```python
from build123d import *

# Parameters (mm, degrees)
F1_DEPTH = 5
F3_DEPTH = 2


with BuildPart() as f1:
    # F0 (on Top) → F1 (new body)
    with BuildSketch(Plane.XY):
        Polygon((37.573822, 49.251007), (-55.58905, 49.251007), (-55.58905, -67.659264), (-31.55629, -43.860067), (37.573822, -43.860067), align=None)
    extrude(amount=F1_DEPTH)

    # F2 (on face) → F3 (cut)
    with BuildSketch(Plane.XY.offset(5)):
        Polygon((-25.10905, 34.337802), (-40.34905, 34.337802), (-40.34905, -27.690759), (-4.78905, -27.690759), (-4.78905, -12.450759), (-25.10905, -12.450759), align=None)
        Polygon((22.333822, 34.337802), (-0.526178, 34.337802), (-13.226178, 19.097802), (7.093822, 19.097802), (7.093822, -27.690759), (22.333822, -27.690759), align=None)
    extrude(amount=-F3_DEPTH, mode=Mode.SUBTRACT)


solid = f1.part
```
Design review of the part built by this model. Coordinates are the model's own, in mm. A direction names the side the tool comes from. Coordinates: 2 decimals unless noted, no trailing zeros. Write each loop counter-clockwise with the first axis right and the second up, starting at its lowest first coordinate (ties: lowest second). Pieces come first, ordered by that corner, then holes.
1) Machinability: for faces 4 (the flat face through (-10, 5, 0)), 5 (the flat face through (-6.79, 26.82, 4.01)), which of the approach directions +Z, -Z, +X, -X, +Y, -Y give a long, thin tool a straight path to every point of the face, cutting with its end or side? Answer none if there is none.
2) Add section A-A (z = 4.2). Write out the cut boundary in (x, y).
3) To check wall thickness, follow L1, parallel to X at y = -24.5, z = 3.75; L2, parallel to X at y = 1, z = 3.75; L3, parallel to Y at x = -9, z = 3.85. State the ranges of each line that lie inside material, in increasing order.
4) Add section D-D (y = -7). Write out the cut boundary in (x, z).
5) Mouldability with a two-part tool opening along Y and no side actions: class faces 1 (the flat face through (-31, -3, 3)), 2 (the flat face through (-8, 49.251, 2)), 3 (the flat face through (3, -43.86, 2)) as +Y half, -Y half, draft (parallel to the pull), parting line (faces both ways), or undercut.
6) Add section C-C (x = 11). Write out the cut boundary in (y, z), plus the area to 3 significant figures.
7) Add section B-B (y = -19). Write out the cut boundary in (x, z), plus the area to 3 significant figures.
8) Insertion check: pin 1 (1 mm diameter, centred on x = 13.5, z = 4, fed in from -Y); pin 2 (0.6 mm diameter, centred on x = -36, z = 4.5, fed in from -Y). Each pin has a flat end and moves straight along its axis. Give the tip position at first contact, or say it passes through.
Check result:
1. face 4: -Z, +X, -X, +Y, -Y
1. face 5: +Z
2. outline: (-55.59, -67.66) - (-31.56, -43.86) - (37.57, -43.86) - (37.57, 49.25) - (-55.59, 49.25) - close; hole (-40.35, -27.69) - (-4.79, -27.69) - (-4.79, -12.45) - (-25.11, -12.45) - (-25.11, 34.34) - (-40.35, 34.34) - close; hole (-13.23, 19.1) - (7.09, 19.1) - (7.09, -27.69) - (22.33, -27.69) - (22.33, 34.34) - (-0.53, 34.34) - close
3. L1: x = -55.59 to -40.35, -4.79 to 7.09, 22.33 to 37.57
3. L2: x = -55.59 to -40.35, -25.11 to 7.09, 22.33 to 37.57
3. L3: y = -43.86 to -27.69, -12.45 to 19.1, 24.17 to 49.25
4. outline: (-55.59, 0) - (37.57, 0) - (37.57, 5) - (22.33, 5) - (22.33, 3) - (7.09, 3) - (7.09, 5) - (-25.11, 5) - (-25.11, 3) - (-40.35, 3) - (-40.35, 5) - (-55.59, 5) - close
5. face 1: undercut
5. face 2: +Y half
5. face 3: -Y half
6. outline: (-43.86, 0) - (49.25, 0) - (49.25, 5) - (34.34, 5) - (34.34, 3) - (-27.69, 3) - (-27.69, 5) - (-43.86, 5) - close
6. area: 341 mm2
7. outline: (-55.59, 0) - (37.57, 0) - (37.57, 5) - (22.33, 5) - (22.33, 3) - (7.09, 3) - (7.09, 5) - (-4.79, 5) - (-4.79, 3) - (-40.35, 3) - (-40.35, 5) - (-55.59, 5) - close
7. area: 364 mm2
8. pin 1: stops at y = -43.86
8. pin 2: stops at y = -48.56
